Geometry: see drawing. Coordinates: mm, zero at the bounding-box minimum. A direction names the side the tool comes from. Give positions to 0.01 mm unless a question says otherwise; leave off trailing zeros. Order: outer loops, then holes, each group sorted by start corner. A loop starts at its lowest first (then second) coordinate and runs counter-clockwise, first axis right, second up. Notation, with made-up numbers: M 34.25,38.5 L 65.25,38.5 A27 cw 65.25,63.5 Z; hole C 24,69 d8. An arc over 180 degrees is marked long. Answer as a JSON object with one key per item and string values. Group by question number.
1. Section query B-B (y = 12.7). Output: boundary loops of the cut face in (x, z) (3 decimals), plus the area to 3 significant figures.
2. Material intervals for L1, parallel to X at y = 12.7, z = 24.6 (3 decimals); L2, parallel to X at y = 12.7, z = 23.25 (3 decimals); L3, parallel to Y at x = 19.05, z = 23.65 (3 decimals), sorted ascending. Write a range as [from, to].
3. Pull-direction query (Y, two-part tool) for the marked faces 1, 2, 3 and 4; classes: +Y half, -Y half, draft (parallel to the pull), parting line (faces both ways), or undercut.
4. Section query C-C (x = 19.05). Output: boundary loops of the cut face in (y, z) (3 decimals), plus the area to 3 significant figures.
5. Section query A-A (z = 12.7). Output: boundary loops of the cut face in (x, y) (3 decimals), plus the area to 3 significant figures.
6. Pin query (flat end, axial travel): P1, Ø12, axis at y = 4.5, z = 15, coming from the -X side; P2, Ø3, axis at y = 12.5, z = 16, coming from the +X side (3 decimals); P3, Ø12, axis at x = 42, y = 9.5, coming from the -Z side (3 decimals); P4, Ø6, axis at y = 22, z = 18, coming from the +X side. Return the tip coordinate at first contact, or that it passes through.
7. Section query D-D (y = 2.75). Output: boundary loops of the cut face in (x, z) (3 decimals).
8. Set-up query: the marked faces 5 and 6. Return all of +Z, -Z, +X, -X, +Y, -Y with unobstructed straight access to the full face (end or side cutting, diameter ignored); none if empty.
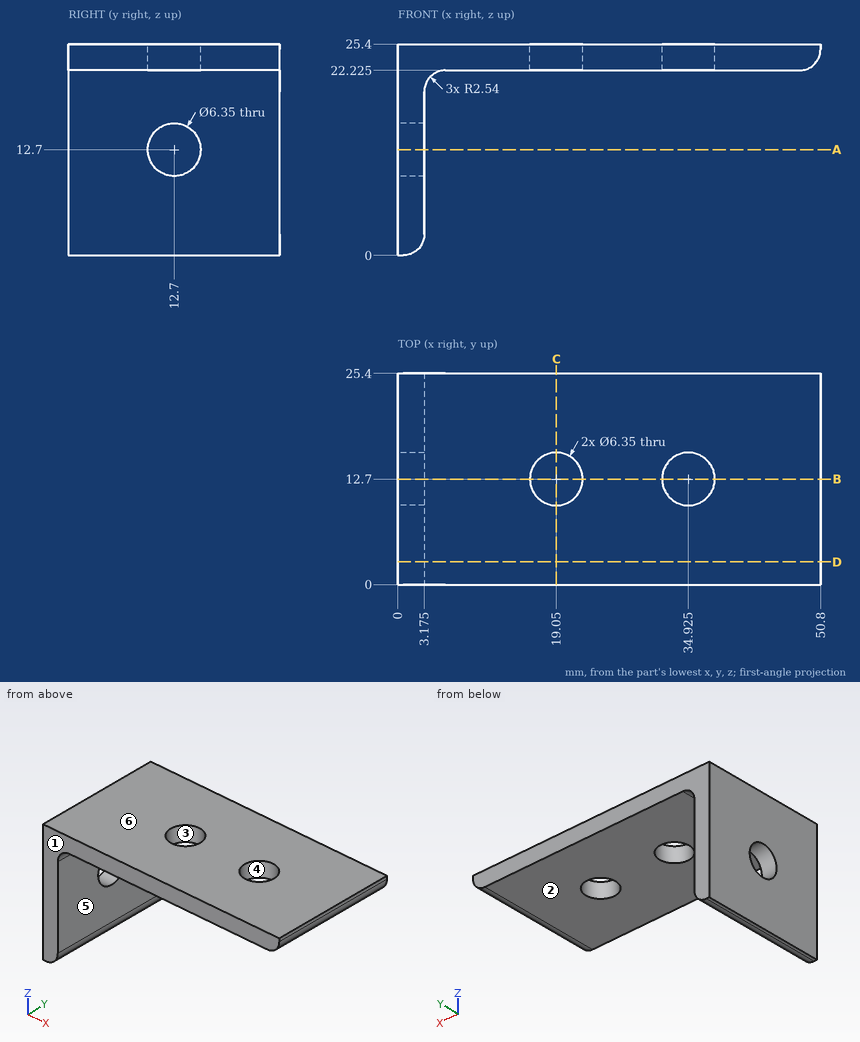
Answer sheet:
{
 "1": {"outline": "M 0,0 L 0.635,0 A2.54 ccw 3.175,2.54 L 3.175,9.525 L 0,9.525 Z; M 0,15.875 L 3.175,15.875 L 3.175,19.685 A2.54 cw 5.715,22.225 L 15.875,22.225 L 15.875,25.4 L 0,25.4 Z; M 22.225,22.225 L 31.75,22.225 L 31.75,25.4 L 22.225,25.4 Z; M 38.1,22.225 L 48.26,22.225 A2.54 ccw 50.8,24.765 L 50.8,25.4 L 38.1,25.4 Z", "area": "170 mm^2"},
 "2": {"L1": "[0, 15.875], [22.225, 31.75], [38.1, 50.795]", "L2": "[0, 15.875], [22.225, 31.75], [38.1, 50.299]", "L3": "[0, 9.525], [15.875, 25.4]"},
 "3": {"face 1": "-Y half", "face 2": "draft", "face 3": "undercut", "face 4": "undercut"},
 "4": {"outline": "M 0,22.225 L 9.525,22.225 L 9.525,25.4 L 0,25.4 Z; M 15.875,22.225 L 25.4,22.225 L 25.4,25.4 L 15.875,25.4 Z", "area": "60.5 mm^2"},
 "5": {"outline": "M 0,0 L 3.175,0 L 3.175,9.525 L 0,9.525 Z; M 0,15.875 L 3.175,15.875 L 3.175,25.4 L 0,25.4 Z", "area": "60.5 mm^2"},
 "6": {"P1": "x = 0", "P2": "x = 3.175", "P3": "z = 22.225", "P4": "x = 3.54"},
 "7": {"outline": "M 0,0 L 0.635,0 A2.54 ccw 3.175,2.54 L 3.175,19.685 A2.54 cw 5.715,22.225 L 48.26,22.225 A2.54 ccw 50.8,24.765 L 50.8,25.4 L 0,25.4 Z"},
 "8": {"face 5": "-Z, +X, +Y, -Y", "face 6": "+Z, +X, -X, +Y, -Y"}
}
